Could you check a few things on this model? Use its own coordinates, in mm. Round coordinates to 2 decimals unless told otherwise and drop trailing zeros. Order: outer loops, then holes, each group sorted by start corner. A loop starts at its lowest first (then second) coordinate and runs counter-clockwise, first axis right, second up. Notation, with made-up numbers: (59.5, -16.75) - (100.5, -16.75) arc R20 cw to (100.5, -10.75) - close; hole circle Ø2 at (55, 71.25). An arc over 180 degrees is marked (long way). Use one line per item in the form item = value.
from build123d import *

# Parameters (mm, degrees)
ESQUISSE1_R        = 4
BOSS_EXTRU_1_DEPTH = 908
FILLET1_R          = 3


with BuildPart() as part:
    # Esquisse1 → Boss.-Extru.1 (new body)
    with BuildSketch(Plane(origin=(1000, 0, 0), x_dir=(0, 0, -1), z_dir=(1, 0, 0))):
        Polygon((22.5, -4), (12.5, -4), (12.5, 4), (22.5, 4), (22.5, 22.5), (4, 22.5), (4, 12.5), (-4, 12.5), (-4, 22.5), (-22.5, 22.5), (-22.5, 4), (-12.5, 4), (-12.5, -4), (-22.5, -4), (-22.5, -22.5), (-4, -22.5), (-4, -12.5), (4, -12.5), (4, -22.5), (22.5, -22.5), align=None)
        Circle(ESQUISSE1_R, mode=Mode.SUBTRACT)
    extrude(amount=-BOSS_EXTRU_1_DEPTH)

    # Fillet1
    fillet1_edges = [part.edges().sort_by_distance(p)[0] for p in [
        (546, -22.5, -22.5),
        (546, -22.5, 22.5),
        (546, 22.5, 22.5),
        (546, 22.5, -22.5),
    ]]
    fillet(fillet1_edges, radius=FILLET1_R)


solid = part.part
Item 1: Will these pins go through, and if not, where does the flat tip stop? P1, Ø8, axis at x = 701, y = 20, coming from the +Z side; P2, Ø2.5, axis at x = 411, y = -1, coming from the +Z side; P3, Ø2.5, axis at x = 622, z = 1.5, coming from the +Y side; P4, Ø2.5, axis at x = 371.5, z = -1.5, coming from the -Y side.
Found:
P1 = 22.5
P2 = 12.5
P3 = 12.5
P4 = -12.5
Item 2: I need wall thicknesses on L1, parallel to Y at x = 413.5, z = -18; L2, parallel to Y at x = 753, z = 0. Which ranges of each line are inside material? Lowest first, please.
Found:
L1 = -22.5 to -4, 4 to 22.5
L2 = -12.5 to -4, 4 to 12.5
Item 3: Imagine slicing it at A-A on x = 147.5. Please give me the cut outline in (y, z).
Found:
outline = (-22.5, -19.5) arc R3 ccw to (-19.5, -22.5) - (-4, -22.5) - (-4, -12.5) - (4, -12.5) - (4, -22.5) - (19.5, -22.5) arc R3 ccw to (22.5, -19.5) - (22.5, -4) - (12.5, -4) - (12.5, 4) - (22.5, 4) - (22.5, 19.5) arc R3 ccw to (19.5, 22.5) - (4, 22.5) - (4, 12.5) - (-4, 12.5) - (-4, 22.5) - (-19.5, 22.5) arc R3 ccw to (-22.5, 19.5) - (-22.5, 4) - (-12.5, 4) - (-12.5, -4) - (-22.5, -4) - close; hole circle Ø8 at (0, 0)
